Part print with two shaded views. Sizes in mm from the minimum x, y, z corner. A direction names the side the tool comes from. Coordinates: 2 decimals unless noted, no trailing zeros. Write each loop counter-clockwise with the first axis right and the second up, starting at its lowest first coordinate (ties: lowest second). Pieces come first, ordered by that corner, then holes. Notation, with made-up numbers: (74.5, -25.5) - (93.5, -25.5) arc R7 cw to (93.5, -16.5) - close; hole circle Ø6 at (3.25, 59.25). An arc over 180 degrees is marked (long way). Answer in a Markdown table with one row per item. Add a question column.
Q1. 3-axis set-ups, long thin cutter, end or side, ignore diameter. For the marked faces 1 and 2: which of +Z, -Z, +X, -X, +Y, -Y reach the whole face in a straight line?
Q2. Band-saw the part on C-C (x = 27.5). List the corners of the cut face in (y, z) (1 decimal).
Q3. Band-saw the part on D-D (z = 69.5). List the corners of the cut face in (x, y).
Q4. Drill centre lines: line 1 along X through (y, z) = (120, 281); line 2 along X through (y, z) = (14.5, 247); line 3 along Y through (x, z) = (81, 221). Where is each one in solid material? Low to high. Write a range as from..to.
Q5. Pin check, flat tips, straight feed: pin 1 (5 mm diameter, centred on y = 40, z = 148, fed in from +X); pin 2 (2 mm diameter, centred on y = 47.5, z = 149.5, fed in from -X) (1 decimal); pin 3 (3 mm diameter, centred on y = 48.5, z = 162.5, fed in from -X). Stop position of each tip, or through.
Q6. Band-saw the part on A-A (y = 14). List the corners of the cut face in (x, z) (1 decimal), and give its area (3 significant figures).
Q7. Two-plate mould, pull along X, no slides. Class the marked faces 3, 4 and 5: +X half, -X half, draft (parallel to the pull), parting line (faces both ways), or undercut.
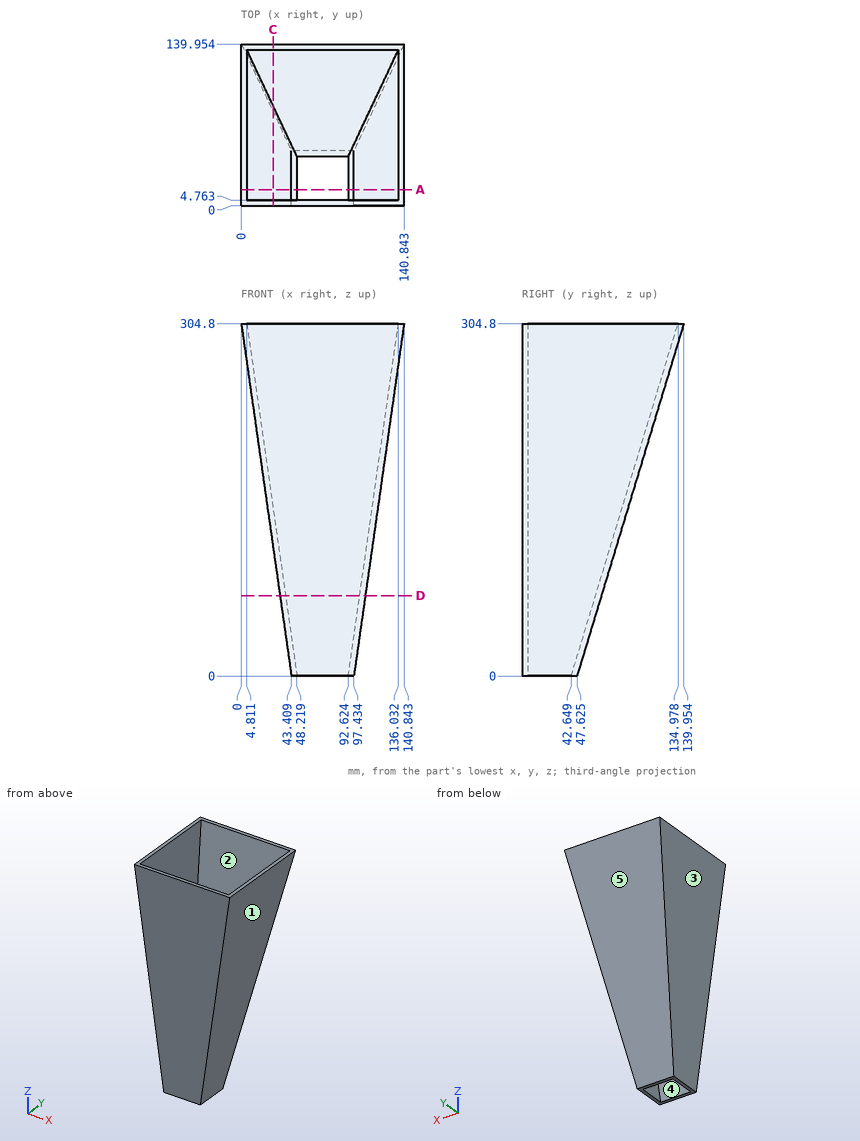
Checked values:
| question | item | result |
|---|---|---|
| 1 | face 1 | -Z, +X, +Y, -Y |
| 1 | face 2 | +Z |
| 2 | outline | (0, 111.7) - (81.5, 111.7) - (140, 304.8) - (135, 304.8) - (86.7, 145.5) - (4.8, 145.5) - (4.8, 304.8) - (0, 304.8) - close |
| 3 | outline | (33.51, 0) - (107.33, 0) - (107.33, 68.68) - (33.51, 68.68) - close; hole (38.32, 4.76) - (102.52, 4.76) - (102.52, 63.7) - (38.32, 63.7) - close |
| 4 | line 1 | x = 3.39..8.2, 132.64..137.45 |
| 4 | line 2 | x = 8.23..13.04, 127.8..132.61 |
| 4 | line 3 | y = 0..4.76, 109.59..114.57 |
| 5 | pin 1 | stops at x = 118.87 |
| 5 | pin 2 | stops at x = 22 |
| 5 | pin 3 | stops at x = 20.05 |
| 6 | outline | (0, 304.8) - (43.4, 0) - (48.2, 0) - (4.8, 304.8) - close; (92.6, 0) - (97.4, 0) - (140.8, 304.8) - (136, 304.8) - close |
| 6 | area | 2,930 mm² |
| 7 | face 3 | -X half |
| 7 | face 4 | undercut |
| 7 | face 5 | draft |
